Could you check a few things on this model? Use its own coordinates, in mm. A direction names the side the tool comes from. Round coordinates to 2 decimals unless told otherwise and drop trailing zeros. Write each loop counter-clockwise with the first axis right and the second up, starting at its lowest first coordinate (ties: lowest second). Pieces come first, ordered by that corner, then holes. Notation, with made-up numbers: (-21, -26.75) -> (29, -26.75) arc R24 ccw to (29, -9.75) -> close; hole circle Ø9 at (-38, 20.25). An arc over 180 degrees is marked (long way). Answer as CSV lines item,"result". Start each with the question number.
Q1. If we mould it in two halves opening along Z, with no side actions, what happens to faces 1 (the cylindrical face through (-15.62, 2.96, -3.47)), 2 (the cylindrical face through (6.69, 3.04, 9)), 3 (the flat face through (0, 0, 0))? For each: pulls with the +Z half, pulls with the -Z half, needs draft (parallel to the pull), parting line crosses it, or undercut.
Q2. Will these pins go through, and if not, where does the flat tip stop? pin 1 Ø5 at (y, z) = (18, -3) entering from +X; pin 2 Ø10 at (y, z) = (3.5, -8.5) entering from -X; pin 3 Ø2 at (x, z) = (10, 12) entering from +Y.
Q3. If I drill on line 1 (Z direction, x = 8, y = 3); line 2 (Y direction, x = 5, z = 6.5), over which ranges is the centre line in solid material (lowest first)? Write a range as [from, to].
Q4. For faces 4 (the flat face through (4, 6, -4)), 5 (the flat face through (0, 30, 0)), which set-ups out of +Z, -Z, +X, -X, +Y, -Y let a thin tool reach every point of the face, with its end or its side?
Q5. Imagine slicing it at A-A on z = -8. Please give me the cut outline in (x, y), and give its area (3 significant figures).
Q6. Imagine slicing it at C-C on x = 2. Please give me the cut outline in (y, z), and give its area (3 significant figures).
Q7. Imagine slicing it at D-D on z = 0. Please give me the cut outline in (x, y).
Q8. Imagine slicing it at B-B on x = 9. Please give me the cut outline in (y, z), and give its area (3 significant figures).
from build123d import *

# Parameters (mm, degrees)
SKETCH1_R                   = 16
BOSS_EXTRUDE1_DEPTH         = 6
TAP_DRILL_FOR_M4X0_7_TAP1_D = 3.3
SKETCH3_R                   = 5
BOSS_EXTRUDE2_DEPTH         = 24


with BuildPart() as part:
    # Sketch1 → Boss-Extrude1 (new body)
    with BuildSketch(Plane(origin=(0, 0, 0), x_dir=(1, 0, 0), z_dir=(0, 1, 0))):
        with Locations(Location((0, 0, 0), (0, 0, 270))):
            Circle(SKETCH1_R)
    extrude(amount=BOSS_EXTRUDE1_DEPTH)

    # Tap Drill for M4x0.7 Tap1 (through all)
    with Locations(Plane(origin=(0, 0, 0), x_dir=(-1, 0, 0), z_dir=(0, -1, 0))):
        with Locations((-8, 8), (-8, -8), (8, -8), (8, 8)):
            Hole(TAP_DRILL_FOR_M4X0_7_TAP1_D / 2)

    # Sketch3 → Boss-Extrude2 (add)
    with BuildSketch(Plane(origin=(0, 6, 0), x_dir=(1, 0, 0), z_dir=(0, 1, 0))):
        with Locations(Location((0, 0, 0), (0, 0, 270))):
            Circle(SKETCH3_R)
    extrude(amount=BOSS_EXTRUDE2_DEPTH)


solid = part.part
Checks:
1,face 1,"parting line crosses it"
1,face 2,"undercut"
1,face 3,"needs draft"
2,pin 1,"x = 4.97"
2,pin 2,"x = -15.61"
2,pin 3,"y = 6"
3,line 1,"[-13.86, -9.65], [-6.35, 6.35], [9.65, 13.86]"
3,line 2,"[0, 6]"
4,face 4,"+Y"
4,face 5,"+Z, -Z, +X, -X, +Y"
5,outline,"(-13.86, 0) -> (-9.65, 0) -> (-9.65, 6) -> (-13.86, 6) -> close; (-6.35, 0) -> (6.35, 0) -> (6.35, 6) -> (-6.35, 6) -> close; (9.65, 0) -> (13.86, 0) -> (13.86, 6) -> (9.65, 6) -> close"
5,area,"127 mm^2"
6,outline,"(0, -15.87) -> (6, -15.87) -> (6, -4.58) -> (30, -4.58) -> (30, 4.58) -> (6, 4.58) -> (6, 15.87) -> (0, 15.87) -> close"
6,area,"410 mm^2"
7,outline,"(-16, 0) -> (16, 0) -> (16, 6) -> (5, 6) -> (5, 30) -> (-5, 30) -> (-5, 6) -> (-16, 6) -> close"
8,outline,"(0, -13.23) -> (6, -13.23) -> (6, -9.31) -> (0, -9.31) -> close; (0, -6.69) -> (6, -6.69) -> (6, 6.69) -> (0, 6.69) -> close; (0, 9.31) -> (6, 9.31) -> (6, 13.23) -> (0, 13.23) -> close"
8,area,"127 mm^2"
